from build123d import *

# Parameters (mm, degrees)
F1_DEPTH = 6.35
F2_R     = 82.87
F3_DEPTH = 6.351
F4_D     = 4.0386
F5_D     = 7.112
F6_D     = 5.1054


with BuildPart() as f1:
    # F0 (on Top) → F1 (new body)
    with BuildSketch(Plane.XY):
        with BuildLine():
            Line((144.6, 170), (-144.6, 170))
            ThreePointArc((-144.6, 170), (-162.5605122421, 162.5605122421), (-170, 144.6))
            Line((-170, 144.6), (-170, -144.6))
            ThreePointArc((-170, -144.6), (-162.5605122421, -162.5605122421), (-144.6, -170))
            Line((-144.6, -170), (144.6, -170))
            ThreePointArc((144.6, -170), (162.5605122421, -162.5605122421), (170, -144.6))
            Line((170, -144.6), (170, 144.6))
            ThreePointArc((170, 144.6), (162.5605122421, 162.5605122421), (144.6, 170))
        make_face()
    extrude(amount=F1_DEPTH)

    # F2 (on face) → F3 (cut, through all)
    with BuildSketch(Plane.XY.offset(6.35)):
        Circle(F2_R)
    extrude(amount=-F3_DEPTH, mode=Mode.SUBTRACT)

    # F4 (through all)
    with Locations(Plane.XY.offset(6.35)):
        with Locations((-152.22, 131.6), (-152.22, 152.22), (-112.55, 152.22), (-112.55, 131.6), (152.22, 131.6), (152.22, 152.22), (112.55, 152.22), (112.55, 131.6), (152.22, -131.6), (152.22, -152.22), (112.55, -152.22), (112.55, -131.6), (-112.55, -152.22), (-112.55, -131.6), (-152.22, -131.6), (-152.22, -152.22)):
            Hole(F4_D / 2)

    # F5 (through all)
    with Locations(Plane.XY.offset(6.35)):
        with Locations((0, 152.4), (152.4, 0), (0, -152.4), (-152.4, 0)):
            Hole(F5_D / 2)

    # F6 (through all)
    with Locations(Plane.XY.offset(6.35)):
        with Locations((-163.65, -116.15), (-163.65, -103.45)):
            Hole(F6_D / 2)


solid = f1.part
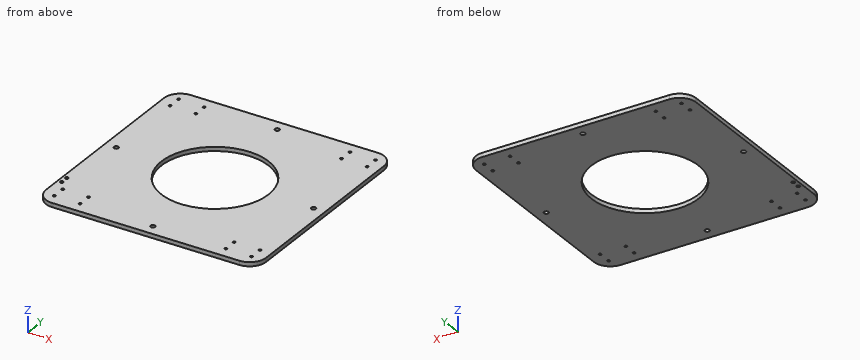
The listing builds one solid part. Answer for the finished solid, in the listing's coordinates (mm). Coordinates: 2 decimals unless noted, no trailing zeros. Loops run counter-clockwise (first coordinate to the right, second up) from the corner with the lowest first, then second, coordinate; pieces in that order, holes last.
1) Flat-ended cylindrical pins translate along their axes: pin 1 Ø3.5 at (x, y) = (152.22, -152.22) entering from -Z; pin 2 Ø3 at (x, y) = (90, 129.5) entering from -Z. Find the tip coordinate at first contact, or state that the pin passes through.
2) Find section C-C on x = 30. Write down the section's boundary in (y, z), then the cut area to 3 significant figures.
3) Find section A-A on y = 12.5. Write down the section's boundary in (x, z).
4) Find section B-B on z = 1. Give the number of separate pieces and of enclosed holes in the cut face, then the cut area to 3 significant figures.
5) Find the intervals of material crossed by L1, parallel to X at y = -131.6, z = 4.75; L2, parallel to Y at x = -112.55, z = 4; L3, parallel to X at y = -152.22, z = 1.5, in increasing order.
Values:
1. pin 1: passes through
1. pin 2: stops at z = 0
2. outline: (-170, 0) - (-77.25, 0) - (-77.25, 6.35) - (-170, 6.35) - close; (77.25, 0) - (170, 0) - (170, 6.35) - (77.25, 6.35) - close
2. area: 1,180 mm2
3. outline: (-170, 0) - (-81.92, 0) - (-81.92, 6.35) - (-170, 6.35) - close; (81.92, 0) - (170, 0) - (170, 6.35) - (81.92, 6.35) - close
4. separate pieces: 1
4. enclosed holes: 23
4. area: 93,100 mm2
5. L1: x = -170 to -154.24, -150.2 to -114.57, -110.53 to 110.53, 114.57 to 150.2, 154.24 to 170
5. L2: y = -170 to -154.24, -150.2 to -133.62, -129.58 to 129.58, 133.62 to 150.2, 154.24 to 170
5. L3: x = -168.83 to -154.24, -150.2 to -114.57, -110.53 to -3.55, 3.55 to 110.53, 114.57 to 150.2, 154.24 to 168.83
